The listing builds one solid part. Answer for the finished solid, in the listing's coordinates (mm). Face numbers are marked on the shaded views. Coordinates: 2 decimals unless noted, no trailing zeros. Loops run counter-clockwise (first coordinate to the right, second up) from the corner with the lowest first, then second, coordinate; pieces in that order, holes last. Notation, with made-up numbers: M 25,25 L 53,25 A18 cw 53,31 Z; hole C -12,50.25 d6. An arc over 180 degrees is marked long. Answer as CSV lines item,"result". Start each with the question number.
```python
from build123d import *

# Parameters (mm, degrees)
F1_DEPTH = 5
F2_R     = 6
F3_DEPTH = 5


with BuildPart() as f1:
    # F0 (on Top) → F1 (new body)
    with BuildSketch(Plane.XY):
        Polygon((0, -62.367893), (0, 19.632107), (-71.014083, -21.367893), align=None)
    extrude(amount=F1_DEPTH)

    # F2 (on face) → F3 (cut, through all)
    with BuildSketch(Plane.XY.offset(5)):
        with Locations((-51.014083, -21.367893)):
            Circle(F2_R)
        with Locations((-30.750196, -34.227709)):
            Circle(F2_R)
        with Locations((-10, -46.287119)):
            Circle(F2_R)
    extrude(amount=-F3_DEPTH, mode=Mode.SUBTRACT)


solid = f1.part
```
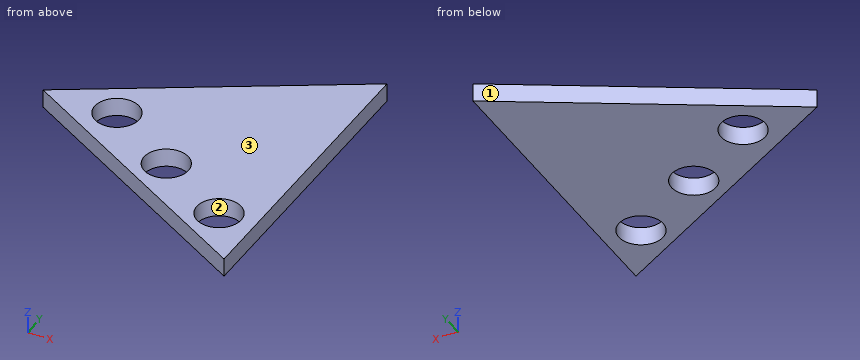
Item 1: For a pull along Y with two mould halves and no side action, classify the marked faces 1, 2 and 3 as pulls with the +Y half, pulls with the -Y half, needs draft (parallel to the pull), parting line crosses it, or undercut.
Item 2: Section B-B on y = -26 is taken. Determine the outline of the cut face in (x, z), then the cut area to 3 significant figures.
Item 3: Consider line 1 (X direction, y = -30, z = 4.4); line 2 (Y direction, x = -54.5, z = 2.3); line 3 (Y direction, x = -15, z = 3.6). Determine where each line is inside the solid, lowest interval first.
Item 4: Each of these flat-tipped pins is pushed along its axis until it touches: P1, Ø3, axis at y = -24, z = 2.5, coming from the +X side; P2, Ø2, axis at x = -57, z = 1.5, coming from the -Y side; P3, Ø1, axis at x = -15.5, z = 0.5, coming from the -Y side; P4, Ø2, axis at x = -24.5, z = 1, coming from the +Y side. Where does it stop, or does it pass through?
Item 5: Section A-A on x = -6.5 is taken. Determine the outline of the cut face in (y, z).
Item 6: Section D-D on y = 13.5 is taken. Determine the outline of the cut face in (x, z).
Item 7: Section C-C on x = -60 is taken. Determine the outline of the cut face in (y, z).
Results are:
1,face 1,"pulls with the +Y half"
1,face 2,"undercut"
1,face 3,"needs draft"
2,outline,"M -62.99,0 L -54.83,0 L -54.83,5 L -62.99,5 Z; M -47.2,0 L 0,0 L 0,5 L -47.2,5 Z"
2,area,"277 mm²"
3,line 1,"-56.06 to -35.01, -26.49 to 0"
3,line 2,"-30.9 to -26.25, -16.48 to -11.83"
3,line 3,"-53.71 to -49.6, -42.97 to 10.97"
4,P1,"x = 0"
4,P2,"y = -30.04"
4,P3,"y = -53.71"
4,P4,"y = 6.06"
5,outline,"M -58.62,0 L -51.16,0 L -51.16,5 L -58.62,5 Z; M -41.41,0 L 15.88,0 L 15.88,5 L -41.41,5 Z"
6,outline,"M -10.62,0 L 0,0 L 0,5 L -10.62,5 Z"
7,outline,"M -27.73,0 L -15.01,0 L -15.01,5 L -27.73,5 Z"
